from build123d import *

# Parameters (mm, degrees)
TORUS_R        = 1.5
CYLINDER_R     = 16
CYLINDER_DEPTH = 50
FILLET001_R    = 1
ARRAY_X_COUNT  = 2
ARRAY_X_PITCH  = 28
ARRAY_Y_COUNT  = 2
ARRAY_Y_PITCH  = 27
BOX_W          = 40
BOX_H          = 40
BOX_DEPTH      = 4
FILLET_R       = 2


with BuildPart() as torus:
    # Torus → Torus (revolve)
    with BuildSketch(Plane(origin=(20, 20, 54), x_dir=(1, 0, 0), z_dir=(0, -1, 0))):
        with Locations((11, 0)):
            Circle(TORUS_R)
    revolve(axis=Axis((20, 20, 54), (0, 0, 1)))


with BuildPart() as cut001:
    # Cylinder → Cylinder (new body)
    with BuildSketch(Plane(origin=(20, 20, 4), x_dir=(1, 0, 0), z_dir=(0, 0, 1))):
        Circle(CYLINDER_R)
    extrude(amount=CYLINDER_DEPTH)

    # Fillet001
    fillet001_edges = [cut001.edges().sort_by_distance(p)[0] for p in [
        (4, 20, 54),
    ]]
    fillet(fillet001_edges, radius=FILLET001_R)

    # Cut001: cut Torus
    add(torus.part, mode=Mode.SUBTRACT)


with BuildPart() as array:
    # Sphere → Sphere (revolve)
    with BuildSketch(Plane(origin=(6, 6, 4), x_dir=(1, 0, 0), z_dir=(0, -1, 0))):
        with BuildLine():
            ThreePointArc((0, -2.4), (2.4, 0), (0, 2.4))
            Line((0, 2.4), (0, -2.4))
        make_face()
    revolve(axis=Axis((6, 6, 4), (0, 0, 1)))

    # Array X: Array ×2


with BuildPart() as array_1:
    add(array.part)
    with Locations(*[(i * ARRAY_X_PITCH, 0, 0) for i in range(1, ARRAY_X_COUNT)]):
        add(array.part)

    # Array Y: Array ×2


with BuildPart() as array_2:
    add(array_1.part)
    with Locations(*[(0, i * ARRAY_Y_PITCH, 0) for i in range(1, ARRAY_Y_COUNT)]):
        add(array_1.part)


with BuildPart() as fusion:
    # Box → Box (new body)
    with BuildSketch(Plane.XY):
        with Locations((20, 20)):
            Rectangle(BOX_W, BOX_H)
    extrude(amount=BOX_DEPTH)

    # Fillet
    fillet_edges = [fusion.edges().sort_by_distance(p)[0] for p in [
        (0, 0, 2),
        (0, 40, 2),
        (40, 0, 2),
        (40, 40, 2),
    ]]
    fillet(fillet_edges, radius=FILLET_R)

    # Cut: cut Array
    add(array_2.part, mode=Mode.SUBTRACT)

    # Fusion: union Cut001
    add(cut001.part)


solid = fusion.part
Model file for the job. Use its own axes, mm. A direction names the side the tool comes from. Give positions to 0.01 mm unless a question says otherwise; leave off trailing zeros. Order: outer loops, then holes, each group sorted by start corner. A loop starts at its lowest first (then second) coordinate and runs counter-clockwise, first axis right, second up. Notation, with made-up numbers: (67.5, -37.5) -> (121.5, -37.5) arc R19 cw to (121.5, -24.5) -> close; hole circle Ø10 at (16, 61.25). An arc over 180 degrees is marked (long way). Use CSV: the item, a comma, the result in double quotes.
1. Drill centre lines: line 1 along Z through (x, y) = (37, 10); line 2 along Z through (x, y) = (18, 5); line 3 along X through (y, z) = (15.5, 25.5). Where is each one in solid material? Low to high. Write a range as from..to.
Outcome:
line 1,"0..4"
line 2,"0..53.99"
line 3,"4.65..35.35"
2. Band-saw the part on A-A, the plane x = 20. Give the cut face in (y, z).
Outcome:
outline,"(0, 0) -> (40, 0) -> (40, 4) -> (36, 4) -> (36, 53) arc R1 ccw to (35, 54) -> (32.5, 54) arc R1.5 cw to (29.5, 54) -> (10.5, 54) arc R1.5 cw to (7.5, 54) -> (5, 54) arc R1 ccw to (4, 53) -> (4, 4) -> (0, 4) -> close"
3. Drop flat-ended pins along their axis: pin 1 (1.5 mm diameter, centred on y = 11.5, z = 16.5, fed in from -X); pin 2 (4 mm diameter, centred on x = 10, z = 46, fed in from +Y); pin 3 (3 mm diameter, centred on x = 36, y = 24.5, fed in from +Z). Give the stop position or say it passes through.
Outcome:
pin 1,"x = 6"
pin 2,"y = 33.86"
pin 3,"z = 53.99"
4. 3-axis set-ups, long thin cutter, end or side, ignore diameter. For faces 1 (the cylindrical face through (0.57, 39.4, 2.03)), 2 (the cylindrical face through (16.53, 4.38, 28.16)): which of +Z, -Z, +X, -X, +Y, -Y reach the whole face in a straight line?
Outcome:
face 1,"+Z, -Z, -X, +Y"
face 2,"+Z"
5. Band-saw the part on B-B, the plane z = 18. Give the cut face in (x, y), then the cut area to 3 significant figures.
Outcome:
outline,"circle Ø32 at (20, 20)"
area,"804 mm²"
